Check sheet for the modelled part. Datum: model origin and axes. Units: mm. Face numbers are marked on the shaded views. A direction names the side the tool comes from. Round coordinates to 2 decimals unless told otherwise and drop trailing zeros. Loops run counter-clockwise (first coordinate to the right, second up) from the corner with the lowest first, then second, coordinate; pieces in that order, holes last. Notation, with made-up numbers: (16.25, -40) - (60.25, -40) arc R13 ccw to (60.25, -31) - close; hole circle Ø10 at (24.5, 78). An arc over 180 degrees is marked (long way). Put each result on its own line as item: value. Start each with the question number.
Item 1: Material ranges on line 1 along Y through (x, z) = (45, 2.5); line 2 along Z through (x, y) = (14, 8); line 3 along Y through (x, z) = (29.5, 3.3), recorded low to high.
Item 2: Draft check along X on the marked faces 1, 2 and 3. Enter one of: pulls with the +X half, pulls with the -X half, needs draft (parallel to the pull), parting line crosses it, or undercut.
Item 3: Section check A-A, the plane z = 1.6. Record the cut outline in (x, y), and give its area (3 significant figures).
Item 4: Gauge pin test, flat ends, axial feed: pin 1 Ø1.8 at (x, y) = (35, 5) entering from +Z; pin 2 Ø0.5 at (x, z) = (28, 3.5) entering from -Y; pin 3 Ø3 at (x, y) = (31.5, 2) entering from +Z; pin 4 Ø0.8 at (x, z) = (41, 3.5) entering from +Y. Record the tip position at first contact, or that the pin passes through.
Item 5: Section check B-B, the plane y = 5. Record the cut outline in (x, z).
Item 6: Tool access check on the marked faces 4 and 5. Record the directions out of +Z, -Z, +X, -X, +Y, -Y that give a thin tool (end or side, any length) a straight path to the whole face; none if there is none.
Item 7: Section check C-C, the plane x = 6. Record the cut outline in (y, z), and give its area (3 significant figures).
from build123d import *

# Parameters (mm, degrees)
ESQUISSE1_W                = 60
ESQUISSE1_H                = 10
BOSS_EXTRU_1_DEPTH         = 3
ESQUISSE2_W                = 60
ESQUISSE2_H                = 2.9
BOSS_EXTRU_2_DEPTH         = 1
ESQUISSE3_R                = 1.5
ENL_V_MAT_EXTRU_1_DEPTH    = 5
R_P_TITION_LIN_AIRE1_COUNT = 6
R_P_TITION_LIN_AIRE1_PITCH = 10


with BuildPart() as part:
    # Esquisse1 → Boss.-Extru.1 (new body)
    with BuildSketch(Plane.XY):
        with Locations((30, 5)):
            Rectangle(ESQUISSE1_W, ESQUISSE1_H)
    extrude(amount=BOSS_EXTRU_1_DEPTH)

    # Esquisse2 → Boss.-Extru.2 (add)
    with BuildSketch(Plane.XY.offset(3)):
        with Locations((30, 5)):
            Rectangle(ESQUISSE2_W, ESQUISSE2_H)
    extrude(amount=BOSS_EXTRU_2_DEPTH)

    # Esquisse3 → Enlèv. mat.-Extru.1 (cut, through all)
    with BuildSketch(Plane(origin=(0, 0, 0), x_dir=(-1, 0, 0), z_dir=(0, 0, -1))):
        with Locations((-55, 5)):
            Circle(ESQUISSE3_R)
    enl_v_mat_extru_1 = extrude(amount=-ENL_V_MAT_EXTRU_1_DEPTH, mode=Mode.SUBTRACT)

    # Répétition linéaire1: Enlèv. mat.-Extru.1 ×6
    with Locations(*[(-i * R_P_TITION_LIN_AIRE1_PITCH, 0, 0) for i in range(1, R_P_TITION_LIN_AIRE1_COUNT)]):
        add(enl_v_mat_extru_1, mode=Mode.SUBTRACT)


solid = part.part
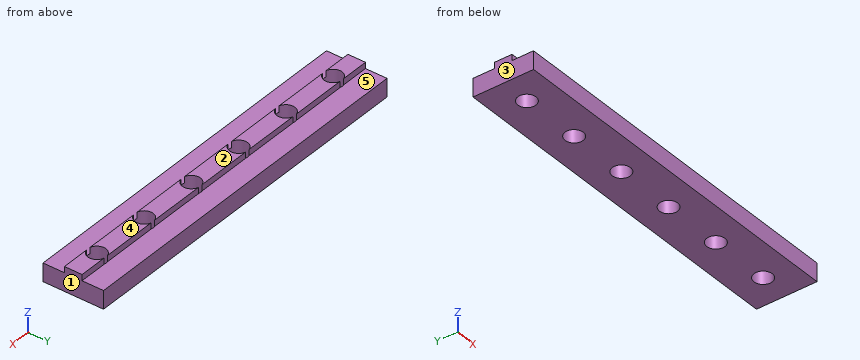
Check result:
1. line 1: 0 to 3.5, 6.5 to 10
1. line 2: 0 to 3
1. line 3: 3.55 to 6.45
2. face 1: pulls with the +X half
2. face 2: needs draft
2. face 3: pulls with the -X half
3. outline: (0, 0) - (60, 0) - (60, 10) - (0, 10) - close; hole circle Ø3 at (5, 5); hole circle Ø3 at (15, 5); hole circle Ø3 at (25, 5); hole circle Ø3 at (35, 5); hole circle Ø3 at (45, 5); hole circle Ø3 at (55, 5)
3. area: 558 mm²
4. pin 1: through
4. pin 2: y = 3.55
4. pin 3: z = 3
4. pin 4: y = 6.45
5. outline: (0, 0) - (3.5, 0) - (3.5, 4) - (0, 4) - close; (6.5, 0) - (13.5, 0) - (13.5, 4) - (6.5, 4) - close; (16.5, 0) - (23.5, 0) - (23.5, 4) - (16.5, 4) - close; (26.5, 0) - (33.5, 0) - (33.5, 4) - (26.5, 4) - close; (36.5, 0) - (43.5, 0) - (43.5, 4) - (36.5, 4) - close; (46.5, 0) - (53.5, 0) - (53.5, 4) - (46.5, 4) - close; (56.5, 0) - (60, 0) - (60, 4) - (56.5, 4) - close
6. face 4: +Z, +X, -X, +Y, -Y
6. face 5: +Z, +X, -X, +Y
7. outline: (0, 0) - (3.88, 0) - (3.88, 4) - (3.55, 4) - (3.55, 3) - (0, 3) - close; (6.12, 0) - (10, 0) - (10, 3) - (6.45, 3) - (6.45, 4) - (6.12, 4) - close
7. area: 24.0 mm²
